```python
from build123d import *

# Parameters (mm, degrees)
F0_R     = 100
F0_R_2   = 75
F1_DEPTH = 120
F2_R     = 95
F2_R_2   = 75
F3_DEPTH = 15
F4_R     = 95
F4_R_2   = 75
F5_DEPTH = 15
F6_R     = 3
F7_DEPTH = 20
F8_R     = 3
F9_DEPTH = 20


with BuildPart() as f1:
    # F0 (on Top) → F1 (new body)
    with BuildSketch(Plane.XY):
        Circle(F0_R)
        Circle(F0_R_2, mode=Mode.SUBTRACT)
    extrude(amount=F1_DEPTH)

    # F2 (on face) → F3 (cut)
    with BuildSketch(Plane.XY.offset(120)):
        Circle(F2_R)
        Circle(F2_R_2, mode=Mode.SUBTRACT)
    extrude(amount=-F3_DEPTH, mode=Mode.SUBTRACT)

    # F4 (on face) → F5 (cut)
    with BuildSketch(Plane(origin=(0, 0, 0), x_dir=(1, 0, 0), z_dir=(0, 0, -1))):
        Circle(F4_R)
        Circle(F4_R_2, mode=Mode.SUBTRACT)
    extrude(amount=-F5_DEPTH, mode=Mode.SUBTRACT)

    # F6 (on face) → F7 (cut)
    with BuildSketch(Plane(origin=(0, 0, 15), x_dir=(1, 0, 0), z_dir=(0, 0, -1))):
        with Locations((85, 0)):
            Circle(F6_R)
        with Locations((-42.5, -73.6121593217)):
            Circle(F6_R)
        with Locations((-42.5, 73.6121593217)):
            Circle(F6_R)
    extrude(amount=-F7_DEPTH, mode=Mode.SUBTRACT)

    # F8 (on face) → F9 (cut)
    with BuildSketch(Plane.XY.offset(105)):
        with Locations((85, 0)):
            Circle(F8_R)
        with Locations((-42.5, -73.6121593217)):
            Circle(F8_R)
        with Locations((-42.5, 73.6121593217)):
            Circle(F8_R)
    extrude(amount=-F9_DEPTH, mode=Mode.SUBTRACT)


solid = f1.part
```
The listing builds one solid part. Answer for the finished solid, in the listing's coordinates (mm). A direction names the side the tool comes from. Coordinates: 2 decimals unless noted, no trailing zeros. Write each loop counter-clockwise with the first axis right and the second up, starting at its lowest first coordinate (ties: lowest second). Pieces come first, ordered by that corner, then holes. Notation, with made-up numbers: (11.5, 26.25) - (26.5, 26.25) arc R22 ccw to (26.5, 59.25) - close; hole circle Ø5 at (-14.75, 1). An arc over 180 degrees is marked (long way). Return JSON: item names as keys, results as strings. Group by question number.
1. Determine the mould class of faces 1 (the flat face through (88, -37, 0)), 2 (the cylindrical face through (82, 0, 95)), 3 (the cylindrical face through (95.38, 30.04, 59.16)) for opening direction X: released by +X, released by -X, zero draft, split by the parting line, or undercut.
2. A cutting plane is placed at D-D, the plane x = 85. Determine the outline of the cut face in (y, z), plus the area to 3 significant figures.
3. Straight lines are drawn through the part: L1, parallel to Y at x = 0, z = 114.75; L2, parallel to Y at x = -42.5, z = 93.25; L3, parallel to Y at x = -47, z = 111.5. For each, find the intervals that lie inside material, in ascending order.
4. A cutting plane is placed at B-B, the plane x = 0. Determine the outline of the cut face in (y, z).
5. Which of the six approach directions +Z, -Z, +X, -X, +Y, -Y give full straight-line access (tool end or side, diameter ignored) to faces 4 (the cylindrical face through (-9.764, 74.362, 59.37)), 5 (the flat face through (-57, -50, 15)), 6 (the flat face through (85, 0, 85))?
6. Given pin 1 (5 mm diameter, centred on x = -30, z = 86.5, fed in from -Y); pin 2 (1.8 mm diameter, centred on x = 85, y = -1, fed in from +Z); pin 3 (1.5 mm diameter, centred on y = -78, z = 104, fed in from +X); pin 4 (3 mm diameter, centred on x = -41.5, y = 59, fed in from +Z), each flat-ended and moving along its own axis, determine where each tip first touches the part or whether it passes through.
7. A cutting plane is placed at A-A, the plane y = 0. Determine the outline of the cut face in (x, z).
8. A cutting plane is placed at C-C, the plane z = 10. Determine the outline of the cut face in (x, y).
Ans:
{
 "1": {"face 1": "zero draft", "face 2": "undercut", "face 3": "split by the parting line"},
 "2": {"outline": "(-52.68, 0) - (-42.43, 0) - (-42.43, 15) - (-3, 15) - (-3, 35) - (3, 35) - (3, 15) - (42.43, 15) - (42.43, 0) - (52.68, 0) - (52.68, 120) - (42.43, 120) - (42.43, 105) - (3, 105) - (3, 85) - (-3, 85) - (-3, 105) - (-42.43, 105) - (-42.43, 120) - (-52.68, 120) - close", "area": "9,860 mm²"},
 "3": {"L1": "-100 to -95, 95 to 100", "L2": "-90.52 to -76.61, -70.61 to -61.8, 61.8 to 70.61, 76.61 to 90.52", "L3": "-88.27 to -82.56, 82.56 to 88.27"},
 "4": {"outline": "(-100, 0) - (-95, 0) - (-95, 15) - (-75, 15) - (-75, 105) - (-95, 105) - (-95, 120) - (-100, 120) - close; (75, 15) - (95, 15) - (95, 0) - (100, 0) - (100, 120) - (95, 120) - (95, 105) - (75, 105) - close"},
 "5": {"face 4": "+Z, -Z", "face 5": "-Z", "face 6": "+Z"},
 "6": {"pin 1": "y = -96.14", "pin 2": "z = 85", "pin 3": "x = 63.5", "pin 4": "through"},
 "7": {"outline": "(-100, 0) - (-95, 0) - (-95, 15) - (-75, 15) - (-75, 105) - (-95, 105) - (-95, 120) - (-100, 120) - close; (75, 15) - (82, 15) - (82, 35) - (88, 35) - (88, 15) - (95, 15) - (95, 0) - (100, 0) - (100, 120) - (95, 120) - (95, 105) - (88, 105) - (88, 85) - (82, 85) - (82, 105) - (75, 105) - close"},
 "8": {"outline": "circle Ø200 at (0, 0); hole circle Ø190 at (0, 0)"}
}
